Model file for the job. Use its own axes, mm. A direction names the side the tool comes from. Coordinates: 2 decimals unless noted, no trailing zeros. Write each loop counter-clockwise with the first axis right and the second up, starting at its lowest first coordinate (ties: lowest second). Pieces come first, ordered by that corner, then holes. Notation, with made-up numbers: M 79.5,86.25 L 91.5,86.25 A21 cw 91.5,94.25 Z; hole C -35.5,1.25 d10. An arc over 180 degrees is marked long. One line per question, with ' | ' between items. Start each with the question number.
(1) Cut at D-D (x = -67.5). Write the cut outline in (y, z).
(2) Cut at B-B (x = 54.5). Write the cut outline in (y, z).
(3) Flat gauge pins, fed straight in: pin 1 Ø2 at (y, z) = (-42, 4.5) entering from +X; pin 2 Ø3 at (x, z) = (-69.5, 4) entering from -Y; pin 3 Ø3.5 at (x, z) = (-82.5, 4.5) entering from -Y. Where does each tip first touch, or does it go through?
(4) Cut at C-C (z = 4.25). Count the separate pieces of the cut face and the enclosed holes in it, plus the area to 3 significant figures.
(5) Two-plate mould, pull along X, no slides. Class faces 1 (the face through (-28.93, -24.42, 3.55)), 2 (the face through (104, -62.126, 4)), 3 (the face through (-60.599, -37, 4)): +X half, -X half, draft (parallel to the pull), parting line (faces both ways), or undercut.
(6) Tool access for faces 4 (the face through (-81, -8.126, 4)), 5 (the face through (142.401, -48, 4)), 6 (the face through (189.62, 82.72, 3.55)): list every direction of +Z, -Z, +X, -X, +Y, -Y with a clear straight run to the whole face (end or side of a thin tool).
(7) Wall check: probe 1 along X at (y, z) = (71, 1); probe 2 along Y at (x, z) = (127, 2.75); probe 3 along X at (y, z) = (-49, 3). Give the ranges that are in metal, low to high.
(8) Cut at A-A (y = 50). Write the cut outline in (x, z), plus the area to 3 significant figures.
from build123d import *

# Parameters (mm, degrees)
SKETCH1_R           = 1.7
SKETCH1_R_2         = 3.175
BOSS_EXTRUDE1_DEPTH = 7


with BuildPart() as part:
    # Sketch1 → Boss-Extrude1 (new body)
    with BuildSketch(Plane.XY.offset(7)):
        with BuildLine():
            Line((100.400666143, -62.126245847), (107.400666143, -62.126245847))
            ThreePointArc((107.400666143, -62.126245847), (110.936200049, -60.661779753), (112.400666143, -57.126245847))
            Line((112.400666143, -57.126245847), (112.400666143, -39.418346536))
            ThreePointArc((112.400666143, -39.418346536), (127.400666143, -24.418346536), (142.400666143, -39.418346536))
            Line((142.400666143, -39.418346536), (142.400666143, -57.126245847))
            ThreePointArc((142.400666143, -57.126245847), (143.865132237, -60.661779753), (147.400666143, -62.126245847))
            Line((147.400666143, -62.126245847), (154.400666143, -62.126245847))
            ThreePointArc((154.400666143, -62.126245847), (157.936200049, -60.661779753), (159.400666143, -57.126245847))
            Line((159.400666143, -57.126245847), (159.400666143, -18.126245847))
            ThreePointArc((159.400666143, -18.126245847), (162.329598331, -11.055178035), (169.400666143, -8.126245847))
            Line((169.400666143, -8.126245847), (189.400666143, -8.126245847))
            ThreePointArc((189.400666143, -8.126245847), (196.471733955, -5.197313659), (199.400666143, 1.873754153))
            Line((199.400666143, 1.873754153), (199.400666143, 72.724252492))
            ThreePointArc((199.400666143, 72.724252492), (189.400666143, 82.724252492), (179.400666143, 72.724252492))
            Line((179.400666143, 72.724252492), (179.400666143, 21.873754153))
            ThreePointArc((179.400666143, 21.873754153), (176.471733955, 14.802686341), (169.400666143, 11.873754153))
            Line((169.400666143, 11.873754153), (-70.599333857, 11.873754153))
            ThreePointArc((-70.599333857, 11.873754153), (-77.670401669, 14.802686341), (-80.599333857, 21.873754153))
            Line((-80.599333857, 21.873754153), (-80.599333857, 72.724252492))
            ThreePointArc((-80.599333857, 72.724252492), (-90.599333857, 82.724252492), (-100.599333857, 72.724252492))
            Line((-100.599333857, 72.724252492), (-100.599333857, 1.873754153))
            ThreePointArc((-100.599333857, 1.873754153), (-97.670401669, -5.197313659), (-90.599333857, -8.126245847))
            Line((-90.599333857, -8.126245847), (-70.599333857, -8.126245847))
            ThreePointArc((-70.599333857, -8.126245847), (-63.528266045, -11.055178035), (-60.599333857, -18.126245847))
            Line((-60.599333857, -18.126245847), (-60.599333857, -57.126245847))
            ThreePointArc((-60.599333857, -57.126245847), (-59.134867763, -60.661779753), (-55.599333857, -62.126245847))
            Line((-55.599333857, -62.126245847), (-48.599333857, -62.126245847))
            ThreePointArc((-48.599333857, -62.126245847), (-45.063799951, -60.661779753), (-43.599333857, -57.126245847))
            Line((-43.599333857, -57.126245847), (-43.599333857, -39.418346536))
            ThreePointArc((-43.599333857, -39.418346536), (-28.599333857, -24.418346536), (-13.599333857, -39.418346536))
            Line((-13.599333857, -39.418346536), (-13.599333857, -57.126245847))
            ThreePointArc((-13.599333857, -57.126245847), (-12.134867763, -60.661779753), (-8.599333857, -62.126245847))
            Line((-8.599333857, -62.126245847), (-1.599333857, -62.126245847))
            ThreePointArc((-1.599333857, -62.126245847), (1.936200049, -60.661779753), (3.400666143, -57.126245847))
            Line((3.400666143, -57.126245847), (3.400666143, -18.126245847))
            ThreePointArc((3.400666143, -18.126245847), (6.329598331, -11.055178035), (13.400666143, -8.126245847))
            Line((13.400666143, -8.126245847), (85.400666143, -8.126245847))
            ThreePointArc((85.400666143, -8.126245847), (92.471733955, -11.055178035), (95.400666143, -18.126245847))
            Line((95.400666143, -18.126245847), (95.400666143, -57.126245847))
            ThreePointArc((95.400666143, -57.126245847), (96.865132237, -60.661779753), (100.400666143, -62.126245847))
        make_face()
        with Locations((-50.189333857, -39.418346536)):
            Circle(SKETCH1_R, mode=Mode.SUBTRACT)
        with Locations((-7.009333857, -39.418346536)):
            Circle(SKETCH1_R, mode=Mode.SUBTRACT)
        with Locations((-28.599333857, -17.066346536)):
            Circle(SKETCH1_R, mode=Mode.SUBTRACT)
        with Locations((-90.599333857, 70.581653464)):
            Circle(SKETCH1_R_2, mode=Mode.SUBTRACT)
        with Locations(Location((189.400666143, 70.581653464, 0), (0, 0, 180))):
            Circle(SKETCH1_R_2, mode=Mode.SUBTRACT)
        with Locations(Location((127.400666143, -17.066346536, 0), (0, 0, 180))):
            Circle(SKETCH1_R, mode=Mode.SUBTRACT)
        with Locations(Location((105.810666143, -39.418346536, 0), (0, 0, 180))):
            Circle(SKETCH1_R, mode=Mode.SUBTRACT)
        with Locations(Location((148.990666143, -39.418346536, 0), (0, 0, 180))):
            Circle(SKETCH1_R, mode=Mode.SUBTRACT)
    extrude(amount=-BOSS_EXTRUDE1_DEPTH)


solid = part.part
Filled in:
1) outline: M -8.62,0 L 11.87,0 L 11.87,7 L -8.62,7 Z
2) outline: M -8.13,0 L 11.87,0 L 11.87,7 L -8.13,7 Z
3) pin 1: x = 159.4 | pin 2: y = -8.47 | pin 3: y = -8.13
4) separate pieces: 1 | enclosed holes: 8 | area: 13,500 mm²
5) face 1: undercut | face 2: draft | face 3: -X half
6) face 4: +Z, -Z, -X, -Y | face 5: +Z, -Z, -Y | face 6: +Z, -Z, +Y
7) probe 1: -100.6 to -93.75, -87.45 to -80.6, 179.4 to 186.25, 192.55 to 199.4 | probe 2: -24.42 to -18.72, -15.41 to 11.87 | probe 3: -60.6 to -43.6, -13.6 to 3.4, 95.4 to 112.4, 142.4 to 159.4
8) outline: M -100.6,0 L -80.6,0 L -80.6,7 L -100.6,7 Z; M 179.4,0 L 199.4,0 L 199.4,7 L 179.4,7 Z | area: 280 mm²
